from build123d import *
from build123d.topology import SkipClean

# Parameters (mm, degrees)
SKETCH1_W           = 39
SKETCH1_H           = 23.712741858
BOSS_EXTRUDE1_DEPTH = 2
SKETCH9_R           = 4.05
CUT_EXTRUDE6_DEPTH  = 5
SKETCH10_R          = 1.25
BOSS_EXTRUDE5_DEPTH = 5.5
SKETCH11_R          = 2.5
CUT_EXTRUDE7_DEPTH  = 5
BOSS_EXTRUDE6_START = -5.5
SKETCH12_R          = 2.5
BOSS_EXTRUDE6_DEPTH = 5.5
BOSS_EXTRUDE7_DEPTH = 28
BOSS_EXTRUDE8_START = 2
SKETCH14_W          = 39
SKETCH14_H          = 29
SKETCH14_R          = 1.25
SKETCH14_R_2        = 4.05
BOSS_EXTRUDE8_DEPTH = 2
SKETCH15_R          = 3
CUT_EXTRUDE8_DEPTH  = 2


with BuildPart() as part:
    # Sketch1 → Boss-Extrude1 (new body)
    with BuildSketch(Plane.XY):
        with Locations((0, -11)):
            Rectangle(SKETCH1_W, SKETCH1_H)
        with BuildLine():
            ThreePointArc((1.25, -19), (0, -17.75), (-1.25, -19))
            ThreePointArc((-1.25, -19), (0, -20.25), (1.25, -19))
        make_face(mode=Mode.SUBTRACT)
        with BuildLine():
            ThreePointArc((-6.75, -11), (-8, -9.75), (-9.25, -11))
            ThreePointArc((-9.25, -11), (-8, -12.25), (-6.75, -11))
        make_face(mode=Mode.SUBTRACT)
        with BuildLine():
            ThreePointArc((1.25, -3), (0, -1.75), (-1.25, -3))
            ThreePointArc((-1.25, -3), (0, -4.25), (1.25, -3))
        make_face(mode=Mode.SUBTRACT)
        with BuildLine():
            ThreePointArc((9.25, -11), (8, -9.75), (6.75, -11))
            ThreePointArc((6.75, -11), (8, -12.25), (9.25, -11))
        make_face(mode=Mode.SUBTRACT)
    extrude(amount=BOSS_EXTRUDE1_DEPTH)

    # Sketch9 → Cut-Extrude6 (cut)
    with BuildSketch(Plane.XY.offset(2)):
        with Locations((0, -11)):
            Circle(SKETCH9_R)
    extrude(amount=-CUT_EXTRUDE6_DEPTH, mode=Mode.SUBTRACT)

    # Sketch10 → Boss-Extrude5 (add)
    # profile 1 of 2: a face of its own
    with BuildSketch(Plane.ZY.offset(19.5)):
        with BuildLine():
            Line((4.2, 3.5), (8.5, 3.5))
            Line((8.5, 3.5), (8.5, 0.5))
            ThreePointArc((8.5, 0.5), (7.474873734, -1.974873734), (5, -3))
            Line((5, -3), (2, -3))
            Line((2, -3), (2, 0.856370929))
            Line((2, 0.856370929), (0, 0.856370929))
            Line((0, 0.856370929), (0, 3.5))
            Line((0, 3.5), (4.2, 3.5))
        make_face()
        with Locations((5.25, 0.25)):
            Circle(SKETCH10_R, mode=Mode.SUBTRACT)
    # profile 2 of 2: a face of its own
    with BuildSketch(Plane.ZY.offset(19.5)):
        with BuildLine():
            Line((5, -19), (2, -19))
            Line((2, -19), (2, -22.856370929))
            Line((2, -22.856370929), (0, -22.856370929))
            Line((0, -22.856370929), (0, -25.5))
            Line((0, -25.5), (4.2, -25.5))
            Line((4.2, -25.5), (8.5, -25.5))
            Line((8.5, -25.5), (8.5, -22.5))
            ThreePointArc((8.5, -22.5), (7.474873734, -20.025126266), (5, -19))
        make_face()
        with Locations((5.25, -22.25)):
            Circle(SKETCH10_R, mode=Mode.SUBTRACT)
    extrude(amount=-BOSS_EXTRUDE5_DEPTH)

    # Sketch11 → Cut-Extrude7 (cut)
    with BuildSketch(Plane.ZY.offset(19.5)):
        with Locations((5.25, 0.25)):
            Circle(SKETCH11_R)
        with Locations(Location((5.25, -22.25, 0), (0, 0, 180))):
            Circle(SKETCH11_R)
    extrude(amount=-CUT_EXTRUDE7_DEPTH, mode=Mode.SUBTRACT)

    # Sketch12 → Boss-Extrude6 (add)
    with BuildSketch(Plane(origin=(19.5, 0, 0), x_dir=(0, 0, -1), z_dir=(1, 0, 0)).offset(BOSS_EXTRUDE6_START)):
        with BuildLine():
            ThreePointArc((-8.5, 0.5), (-7.474873734, -1.974873734), (-5, -3))
            Line((-5, -3), (-2, -3))
            Line((-2, -3), (-2, -19))
            Line((-2, -19), (-5, -19))
            ThreePointArc((-5, -19), (-7.474873734, -20.025126266), (-8.5, -22.5))
            Line((-8.5, -22.5), (-8.5, -25.5))
            Line((-8.5, -25.5), (0, -25.5))
            Line((0, -25.5), (0, 3.5))
            Line((0, 3.5), (-8.5, 3.5))
            Line((-8.5, 3.5), (-8.5, 0.5))
        make_face()
        with Locations((-5.25, -22.25)):
            Circle(SKETCH12_R, mode=Mode.SUBTRACT)
        with Locations(Location((-5.25, 0.25, 0), (0, 0, 180))):
            Circle(SKETCH12_R, mode=Mode.SUBTRACT)
    extrude(amount=BOSS_EXTRUDE6_DEPTH)

    # Sketch13 → Boss-Extrude7 (add)
    with BuildSketch(Plane.ZY.offset(-14)):
        Polygon((0, 3.5), (4.2, 3.5), (2, 1.3), (2, 0.856370929), (0, 0.856370929), align=None)
        Polygon((2, -22.856370929), (0, -22.856370929), (0, -25.5), (4.2, -25.5), (2, -23.3), align=None)
    extrude(amount=BOSS_EXTRUDE7_DEPTH)

    # Sketch14 → Boss-Extrude8 (add)
    with SkipClean():  # the faces are left unmerged after this step: merging them gives an invalid solid
        with BuildSketch(Plane(origin=(0, 0, 0), x_dir=(-1, 0, 0), z_dir=(0, 0, -1)).offset(BOSS_EXTRUDE8_START)):
            with Locations((0, -11)):
                Rectangle(SKETCH14_W, SKETCH14_H)
            with Locations((0, -19)):
                Circle(SKETCH14_R, mode=Mode.SUBTRACT)
            with Locations((8, -11)):
                Circle(SKETCH14_R, mode=Mode.SUBTRACT)
            with Locations((0, -3)):
                Circle(SKETCH14_R, mode=Mode.SUBTRACT)
            with Locations(Location((0, -11, 0), (0, 0, 180))):
                Circle(SKETCH14_R_2, mode=Mode.SUBTRACT)
            with Locations((-8, -11)):
                Circle(SKETCH14_R, mode=Mode.SUBTRACT)
        extrude(amount=-BOSS_EXTRUDE8_DEPTH)

    # Sketch15 → Cut-Extrude8 (cut)
    with BuildSketch(Plane.XY.offset(2)):
        with Locations((0, -3)):
            Circle(SKETCH15_R)
        with Locations((8, -11)):
            Circle(SKETCH15_R)
        with Locations((0, -19)):
            Circle(SKETCH15_R)
        with Locations((-8, -11)):
            Circle(SKETCH15_R)
    extrude(amount=-CUT_EXTRUDE8_DEPTH, mode=Mode.SUBTRACT)


solid = part.part
Part model, mm, in its own coordinate system. A direction names the side the tool comes from. Coordinates: 2 decimals unless noted, no trailing zeros. Loops run counter-clockwise (first coordinate to the right, second up) from the corner with the lowest first, then second, coordinate; pieces in that order, holes last. Notation, with made-up numbers: (68.5, 85.25) -> (90.5, 85.25) arc R21 ccw to (90.5, 97.25) -> close; hole circle Ø4 at (79.25, 34). An arc over 180 degrees is marked (long way). Use a Markdown table: item, result. Add a question column.
Item 1: Which spindle directions (+Z, -Z, +X, -X, +Y, -Y) get a long thin tool onto all of the face, cutting with end or side? Do faces 5 (the cylindrical face through (-16.79, -20.05, 7.5)), 6 (the cylindrical face through (-0.65, -5.93, 1.01)), 7 (the cylindrical face through (16.71, -20.14, 3.91)). Say none if no direction does.
Item 2: Band-saw the part on C-C on z = -0.5. Write the cut outline in (x, y), plus the area to 3 significant figures.
Item 3: Probe probe 1 along Y at (x, z) = (0, 0.5); probe 2 along Y at (x, z) = (0, -0.6); probe 3 along X at (y, z) = (-19.25, 3.5). List the from-to ranges inside material, lowest first.
Item 4: Band-saw the part on B-B on y = -11. Write the cut outline in (x, z).
Item 5: Band-saw the part on D-D on x = -15. Write the cut outline in (y, z).
Item 6: Band-saw the part on A-A on x = 0. Write the cut outline in (y, z).
Item 7: Pull direction Z, two halves, no side cores. Call faces 1 (the cylindrical face through (-14.3, 0.3, 4)), 2 (the cylindrical face through (16.712, -0.501, 7.635)), 3 (the flat face through (17, -24, 8.5)), 4 (the flat face through (-17, -19, 4)): +Z half, -Z half, draft (parallel to the pull), parting line (faces both ways), or undercut.
Item 8: Flat gauge pins, fed straight in: P1, Ø1.8, axis at x = 0, y = -19.5, coming from the +Z side; P2, Ø6.5, axis at x = 9, y = -12.5, coming from the +Z side; P3, Ø3, axis at y = 0.25, z = 5.25, coming from the -X side. Where does each tip first touch, or does it go through?
Geometry says:
| question | item | result |
|---|---|---|
| 1 | face 5 | +Z, +X, -X |
| 1 | face 6 | +Z |
| 1 | face 7 | +X |
| 2 | outline | (-19.5, -25.5) -> (19.5, -25.5) -> (19.5, 3.5) -> (-19.5, 3.5) -> close; hole circle Ø2.5 at (-8, -11); hole circle Ø8.1 at (0, -11); hole circle Ø2.5 at (0, -19); hole circle Ø2.5 at (0, -3); hole circle Ø2.5 at (8, -11) |
| 2 | area | 1,060 mm² |
| 3 | probe 1 | -25.5 to -22, -16 to -15.05, -6.95 to -6, 0 to 3.5 |
| 3 | probe 2 | -25.5 to -20.25, -17.75 to -15.05, -6.95 to -4.25, -1.75 to 3.5 |
| 3 | probe 3 | -19.5 to -14, 14 to 19.5 |
| 4 | outline | (-19.5, -2) -> (-9.25, -2) -> (-9.25, 0) -> (-11, 0) -> (-11, 2) -> (-19.5, 2) -> close; (-6.75, -2) -> (-4.05, -2) -> (-4.05, 2) -> (-5, 2) -> (-5, 0) -> (-6.75, 0) -> close; (4.05, -2) -> (6.75, -2) -> (6.75, 0) -> (5, 0) -> (5, 2) -> (4.05, 2) -> close; (9.25, -2) -> (19.5, -2) -> (19.5, 2) -> (11, 2) -> (11, 0) -> (9.25, 0) -> close |
| 5 | outline | (-25.5, -2) -> (3.5, -2) -> (3.5, 8.5) -> (0.5, 8.5) arc R3.5 ccw to (-3, 5) -> (-3, 2) -> (-19, 2) -> (-19, 5) arc R3.5 ccw to (-22.5, 8.5) -> (-25.5, 8.5) -> close; hole circle Ø5 at (-22.25, 5.25); hole circle Ø5 at (0.25, 5.25) |
| 6 | outline | (-25.5, -2) -> (-20.25, -2) -> (-20.25, 0) -> (-22, 0) -> (-22, 2) -> (-23.3, 2) -> (-25.5, 4.2) -> close; (-17.75, -2) -> (-15.05, -2) -> (-15.05, 2) -> (-16, 2) -> (-16, 0) -> (-17.75, 0) -> close; (-6.95, -2) -> (-4.25, -2) -> (-4.25, 0) -> (-6, 0) -> (-6, 2) -> (-6.95, 2) -> close; (-1.75, -2) -> (3.5, -2) -> (3.5, 4.2) -> (1.3, 2) -> (0, 2) -> (0, 0) -> (-1.75, 0) -> close |
| 7 | face 1 | undercut |
| 7 | face 2 | undercut |
| 7 | face 3 | +Z half |
| 7 | face 4 | draft |
| 8 | P1 | z = 0 |
| 8 | P2 | z = 2 |
| 8 | P3 | x = -14.5 |
